from build123d import *

# Parameters (mm, degrees)
SKETCH2_W                         = 54
SKETCH2_H                         = 162
SKETCH2_R                         = 10.5
BOSS_EXTRUDE1_DEPTH               = 12
SKETCH3_W                         = 18
SKETCH3_H                         = 12
BOSS_EXTRUDE2_DEPTH               = 12
CUT_EXTRUDE1_REACH                = 99.581
SKETCH4_R                         = 2.25
LPATTERN1_COUNT                   = 2
LPATTERN1_PITCH                   = 90
CUT_EXTRUDE2_DEPTH                = 6
CUT_EXTRUDE3_REACH                = 99.581
SKETCH6_W                         = 24
SKETCH6_H                         = 20
CUT_EXTRUDE4_REACH                = 99.581
SKETCH7_R                         = 3
CUT_EXTRUDE5_DEPTH                = 6
CUT_EXTRUDE6_REACH                = 99.581
SKETCH9_R                         = 5
HOLE1_D                           = 6
HOLE1_CBORE_D                     = 10
HOLE1_CBORE_DEPTH                 = 6
F_6_0_6_DIAMETER_HOLE1_AT_2_COUNT = 2
F_6_0_6_DIAMETER_HOLE1_AT_2_PITCH = 36


with BuildPart() as part:
    # Sketch2 → Boss-Extrude1 (new body)
    with BuildSketch(Plane(origin=(0, 0, 0), x_dir=(0, 0, -1), z_dir=(1, 0, 0))):
        Rectangle(SKETCH2_W, SKETCH2_H)
        Circle(SKETCH2_R, mode=Mode.SUBTRACT)
        with Locations((0, 45)):
            Circle(SKETCH2_R, mode=Mode.SUBTRACT)
        with Locations((0, -45)):
            Circle(SKETCH2_R, mode=Mode.SUBTRACT)
    extrude(amount=BOSS_EXTRUDE1_DEPTH)

    # Sketch3 → Boss-Extrude2 (add)
    with BuildSketch(Plane(origin=(12, 0, 0), x_dir=(0, 0, -1), z_dir=(1, 0, 0))):
        with Locations((0, -87)):
            Rectangle(SKETCH3_W, SKETCH3_H)
    boss_extrude2 = extrude(amount=-BOSS_EXTRUDE2_DEPTH)

    # Mirror1: Boss-Extrude2 across plane
    add(boss_extrude2.mirror(Plane.ZX))

    # Sketch4 → Cut-Extrude1 (cut, up to next)
    with BuildSketch(Plane(origin=(12, 0, 0), x_dir=(0, 0, -1), z_dir=(1, 0, 0)), mode=Mode.PRIVATE) as cut_extrude1_sk1:
        with Locations((-16, -45)):
            Circle(SKETCH4_R)
    cut_extrude1_tool1 = extrude(cut_extrude1_sk1.sketch, amount=-CUT_EXTRUDE1_REACH, mode=Mode.PRIVATE) & part.part
    # Sketch4 → Cut-Extrude1 (cut, up to next)
    with BuildSketch(Plane(origin=(12, 0, 0), x_dir=(0, 0, -1), z_dir=(1, 0, 0)), mode=Mode.PRIVATE) as cut_extrude1_sk2:
        with Locations((16, -45)):
            Circle(SKETCH4_R)
    cut_extrude1_tool2 = extrude(cut_extrude1_sk2.sketch, amount=-CUT_EXTRUDE1_REACH, mode=Mode.PRIVATE) & part.part
    cut_extrude1_1 = cut_extrude1_tool1.solids().sort_by_distance((12, -45, 16))[0]
    add(cut_extrude1_1, mode=Mode.SUBTRACT)
    cut_extrude1_2 = cut_extrude1_tool2.solids().sort_by_distance((12, -45, -16))[0]
    add(cut_extrude1_2, mode=Mode.SUBTRACT)
    cut_extrude1 = cut_extrude1_1 + cut_extrude1_2  # Cut-Extrude1 as one shape, for the pattern or mirror that repeats it

    # LPattern1: Cut-Extrude1 ×2
    with Locations(*[(0, i * LPATTERN1_PITCH, 0) for i in range(1, LPATTERN1_COUNT)]):
        add(cut_extrude1, mode=Mode.SUBTRACT)

    # Sketch5 → Cut-Extrude2 (cut)
    with BuildSketch(Plane.ZY):
        with BuildLine():
            Line((-16.992645468, 60.5), (16.992645468, 60.5))
            ThreePointArc((16.992645468, 60.5), (23, 45), (16.992645468, 29.5))
            Line((16.992645468, 29.5), (-16.992645468, 29.5))
            ThreePointArc((-16.992645468, 29.5), (-23, 45), (-16.992645468, 60.5))
        make_face()
        with BuildLine():
            Line((-16.992645468, -29.5), (16.992645468, -29.5))
            ThreePointArc((16.992645468, -29.5), (23, -45), (16.992645468, -60.5))
            Line((16.992645468, -60.5), (-16.992645468, -60.5))
            ThreePointArc((-16.992645468, -60.5), (-23, -45), (-16.992645468, -29.5))
        make_face()
    extrude(amount=-CUT_EXTRUDE2_DEPTH, mode=Mode.SUBTRACT)

    # Sketch6 → Cut-Extrude3 (cut, up to next)
    with BuildSketch(Plane.ZY, mode=Mode.PRIVATE) as cut_extrude3_sk1:
        with Locations((27, 0)):
            Rectangle(SKETCH6_W, SKETCH6_H)
    cut_extrude3_tool1 = extrude(cut_extrude3_sk1.sketch, amount=-CUT_EXTRUDE3_REACH, mode=Mode.PRIVATE) & part.part
    add(cut_extrude3_tool1.solids().sort_by_distance((0, 0, 27))[0], mode=Mode.SUBTRACT)

    # Sketch7 → Cut-Extrude4 (cut, up to next)
    with BuildSketch(Plane.ZY, mode=Mode.PRIVATE) as cut_extrude4_sk1:
        with Locations((21, 22.5)):
            Circle(SKETCH7_R)
    cut_extrude4_tool1 = extrude(cut_extrude4_sk1.sketch, amount=-CUT_EXTRUDE4_REACH, mode=Mode.PRIVATE) & part.part
    # Sketch7 → Cut-Extrude4 (cut, up to next)
    with BuildSketch(Plane.ZY, mode=Mode.PRIVATE) as cut_extrude4_sk2:
        with Locations((21, -22.5)):
            Circle(SKETCH7_R)
    cut_extrude4_tool2 = extrude(cut_extrude4_sk2.sketch, amount=-CUT_EXTRUDE4_REACH, mode=Mode.PRIVATE) & part.part
    add(cut_extrude4_tool1.solids().sort_by_distance((0, 22.5, 21))[0], mode=Mode.SUBTRACT)
    add(cut_extrude4_tool2.solids().sort_by_distance((0, -22.5, 21))[0], mode=Mode.SUBTRACT)

    # Sketch8 → Cut-Extrude5 (cut)
    with BuildSketch(Plane.ZY):
        with BuildLine():
            Line((21, 27.5), (27, 27.5))
            Line((27, 27.5), (27, 17.5))
            Line((27, 17.5), (21, 17.5))
            ThreePointArc((21, 17.5), (16, 22.5), (21, 27.5))
        make_face()
        with BuildLine():
            Line((21, -27.5), (27, -27.5))
            Line((27, -27.5), (27, -17.5))
            Line((27, -17.5), (21, -17.5))
            ThreePointArc((21, -17.5), (16, -22.5), (21, -27.5))
        make_face()
    extrude(amount=-CUT_EXTRUDE5_DEPTH, mode=Mode.SUBTRACT)

    # Sketch9 → Cut-Extrude6 (cut, up to next)
    with BuildSketch(Plane.ZY, mode=Mode.PRIVATE) as cut_extrude6_sk1:
        with Locations((-18, -69)):
            Circle(SKETCH9_R)
    cut_extrude6_tool1 = extrude(cut_extrude6_sk1.sketch, amount=-CUT_EXTRUDE6_REACH, mode=Mode.PRIVATE) & part.part
    # Sketch9 → Cut-Extrude6 (cut, up to next)
    with BuildSketch(Plane.ZY, mode=Mode.PRIVATE) as cut_extrude6_sk2:
        with Locations((18, -69)):
            Circle(SKETCH9_R)
    cut_extrude6_tool2 = extrude(cut_extrude6_sk2.sketch, amount=-CUT_EXTRUDE6_REACH, mode=Mode.PRIVATE) & part.part
    cut_extrude6_1 = cut_extrude6_tool1.solids().sort_by_distance((0, -69, -18))[0]
    add(cut_extrude6_1, mode=Mode.SUBTRACT)
    cut_extrude6_2 = cut_extrude6_tool2.solids().sort_by_distance((0, -69, 18))[0]
    add(cut_extrude6_2, mode=Mode.SUBTRACT)
    cut_extrude6 = cut_extrude6_1 + cut_extrude6_2  # Cut-Extrude6 as one shape, for the pattern or mirror that repeats it

    # Hole1 (through all)
    with Locations(Plane.ZY):
        with Locations((0, -87)):
            hole1 = CounterBoreHole(HOLE1_D / 2, HOLE1_CBORE_D / 2, HOLE1_CBORE_DEPTH)

    # Sketch13 → Ø6.0 (6) Diameter Hole1 (revolve, cut)
    with BuildSketch(Plane(origin=(6, -81, -18), x_dir=(0, 0, -1), z_dir=(1, 0, 0))):
        Polygon((0, 0), (0, 20.802581857), (3, 19), (3, 0), align=None)
    f_6_0_6_diameter_hole1 = revolve(axis=Axis((6, -87.35, -18), (0, 1, 0)), mode=Mode.SUBTRACT)

    # Ø6.0 (6) Diameter Hole1 at 2: Ø6.0 (6) Diameter Hole1 ×2
    with Locations(*[(0, 0, i * F_6_0_6_DIAMETER_HOLE1_AT_2_PITCH) for i in range(1, F_6_0_6_DIAMETER_HOLE1_AT_2_COUNT)]):
        add(f_6_0_6_diameter_hole1, mode=Mode.SUBTRACT)

    # Mirror2: Cut-Extrude6, Hole1, Ø6.0 (6) Diameter Hole1 across plane
    add(cut_extrude6.mirror(Plane.ZX), mode=Mode.SUBTRACT)
    add(hole1.mirror(Plane.ZX), mode=Mode.SUBTRACT)
    add(f_6_0_6_diameter_hole1.mirror(Plane.ZX), mode=Mode.SUBTRACT)

    # Mirror2 copy 1 sketch → Mirror2 copy 1 (revolve, cut)
    with BuildSketch(Plane(origin=(6, 81, 18), x_dir=(0, 0, -1), z_dir=(1, 0, 0))):
        Polygon((0, 0), (0, -20.802581857), (3, -19), (3, 0), align=None)
    revolve(axis=Axis((6, 87.35, 18), (0, 1, 0)), mode=Mode.SUBTRACT)


solid = part.part
For this review, take the finished solid that the model builds, in its own axes (mm). A direction names the side the tool comes from. Round coordinates to 2 decimals unless told otherwise and drop trailing zeros. Loops run counter-clockwise (first coordinate to the right, second up) from the corner with the lowest first, then second, coordinate; pieces in that order, holes last. Notation, with made-up numbers: (-30, 1) - (5, 1) arc R23 cw to (5, 25) - close; hole circle Ø5 at (24, 32). An arc over 180 degrees is marked (long way). Put each result on its own line as item: value. Start each with the question number.
1. For probe 1 along Y at (x, z) = (3, 12); probe 2 along Z at (x, y) = (6, 63.85); probe 3 along Y at (x, z) = (1.75, 0), list the stretches that pass through material, from the lowest coordinate up. Write a range as [from, to].
2. Consider section D-D on y = -22.5. State the section outline as (x, z) points, plus the area to 3 significant figures.
3. For faces 1 (the flat face through (6, -87, -9)), 2 (the cylindrical face through (3, -45, 23)), 3 (the flat face through (6, 21, 24)), list the 3-axis set-ups (+Z, -Z, +X, -X, +Y, -Y) from which the entire face can be reached by the end or side of a thin tool; tool diameter is ignored.
4. Mouldability with a two-part tool opening along X and no side actions: class faces 4 (the flat face through (3, 29.5, 0)), 5 (the cylindrical face through (7.15, 63.19, 15.23)), 6 (the flat face through (12, 1, -12)) as +X half, -X half, draft (parallel to the pull), parting line (faces both ways), or undercut.
5. Insertion check: P1, Ø1, axis at x = 2.5, z = -10, coming from the +Y side; P2, Ø5, axis at y = 40.5, z = 13.5, coming from the -X side; P3, Ø6, axis at x = 5, y = -86, coming from the -Z side. Each pin has a flat end and moves straight along its axis. Give the tip position at first contact, or say it passes through.
6. Consider section C-C on z = 0. State how many separate pieces and enclosed holes the cut face has, plus the area to 3 significant figures.
7. Consider section A-A on y = 87. State the section outline as (x, z) points, plus the area to 3 significant figures.
8. Consider section B-B on y = -69. State the section outline as (x, z) points.
Result sheet:
1. probe 1: [-81, -60.5], [-29.5, 29.5], [60.5, 81]
1. probe 2: [-27, -21], [-15, 15], [21, 27]
1. probe 3: [-93, -92], [-82, -60.5], [-29.5, -10.5], [10.5, 29.5], [60.5, 82], [92, 93]
2. outline: (0, -27) - (12, -27) - (12, 18) - (6, 18) - (6, 16) - (0, 16) - close; (6, 24) - (12, 24) - (12, 27) - (6, 27) - close
2. area: 546 mm^2
3. face 1: -Z, +X, -X, -Y
3. face 2: -X
3. face 3: +Z, -X
4. face 4: draft
4. face 5: undercut
4. face 6: +X half
5. P1: y = 81
5. P2: x = 6
5. P3: z = -9
6. separate pieces: 6
6. enclosed holes: 0
6. area: 1,160 mm^2
7. outline: (0, -9) - (12, -9) - (12, -3) - (6, -3) - (6, -5) - (0, -5) - close; (0, 5) - (6, 5) - (6, 3) - (12, 3) - (12, 9) - (0, 9) - close
7. area: 120 mm^2
8. outline: (0, -27) - (12, -27) - (12, -23) - (0, -23) - close; (0, -13) - (12, -13) - (12, 13) - (0, 13) - close; (0, 23) - (12, 23) - (12, 27) - (0, 27) - close
